Input: dimensioned drawing with shaded views. Units: mm. Origin: part minimum x, y, z. Give positions to 0.01 mm unless a question says otherwise; leave off trailing zeros. Write each loop counter-clockwise with the first axis right and the second up, starting at its lowest first coordinate (ties: lowest second). Pieces come first, ordered by that corner, then holes.
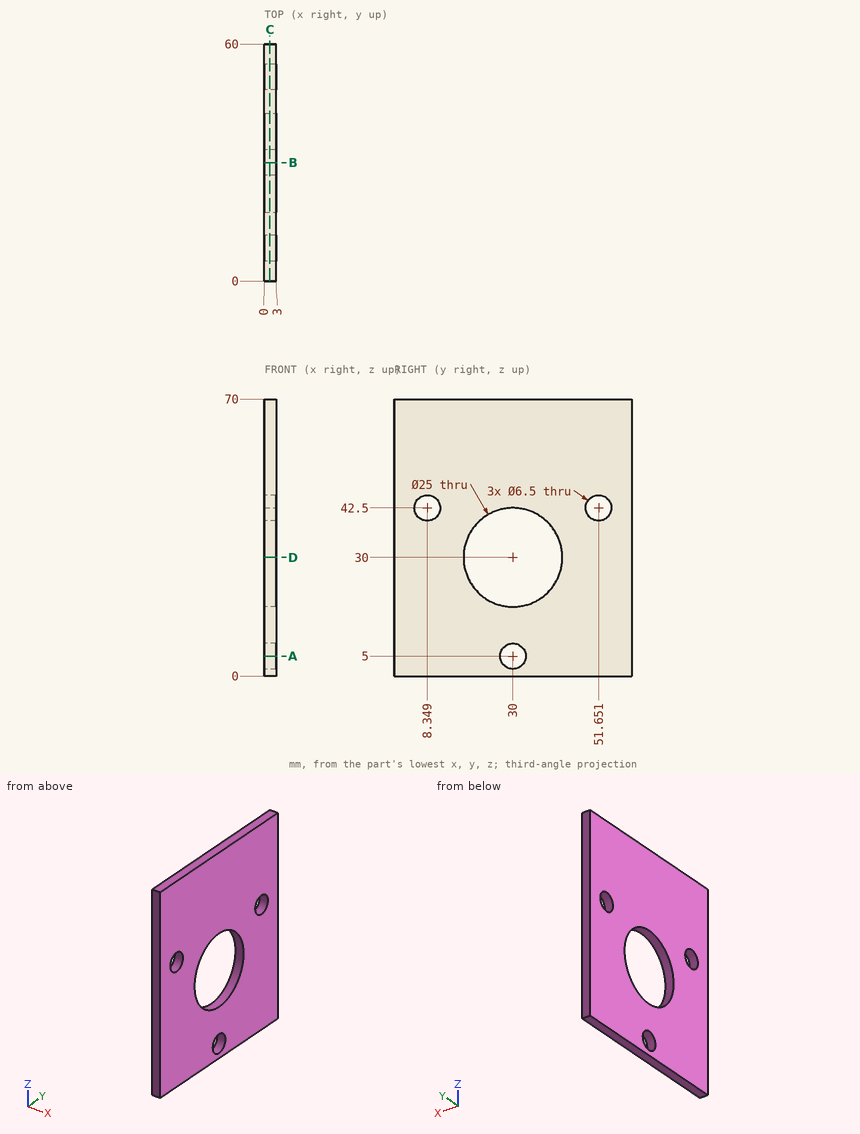
1. Contact query for a flat-ended pin moving along its axis: P1, Ø8.5, axis at y = 8.35, z = 42.5, coming from the -X side. Output: stop coordinate, or through.
2. Cut plane B-B, the plane y = 30. Return the cut outline in (x, z).
3. Cut plane A-A, the plane z = 5. Return the cut outline in (x, y).
4. Cut plane D-D, the plane z = 30. Return the cut outline in (x, y).
5. Line query: L1, parallel to Y at x = 0.5, z = 30.5; L2, parallel to Z at x = 1.95, y = 28.5; L3, parallel to Z at x = 2.35, y = 29. Output: solid intervals per line, ascending.
6. Cut plane C-C, the plane x = 1.4. Return the cut outline in (y, z), then the cut area to 3 significant figures.
Response values:
1. P1: stops at x = 0
2. outline: (0, 0) - (3, 0) - (3, 1.75) - (0, 1.75) - close; (0, 8.25) - (3, 8.25) - (3, 17.5) - (0, 17.5) - close; (0, 42.5) - (3, 42.5) - (3, 70) - (0, 70) - close
3. outline: (0, 0) - (3, 0) - (3, 26.75) - (0, 26.75) - close; (0, 33.25) - (3, 33.25) - (3, 60) - (0, 60) - close
4. outline: (0, 0) - (3, 0) - (3, 17.5) - (0, 17.5) - close; (0, 42.5) - (3, 42.5) - (3, 60) - (0, 60) - close
5. L1: y = 0 to 17.51, 42.49 to 60
5. L2: z = 0 to 2.12, 7.88 to 17.59, 42.41 to 70
5. L3: z = 0 to 1.91, 8.09 to 17.54, 42.46 to 70
6. outline: (0, 0) - (60, 0) - (60, 70) - (0, 70) - close; hole circle Ø6.5 at (8.35, 42.5); hole circle Ø25 at (30, 30); hole circle Ø6.5 at (30, 5); hole circle Ø6.5 at (51.65, 42.5)
6. area: 3,610 mm2
